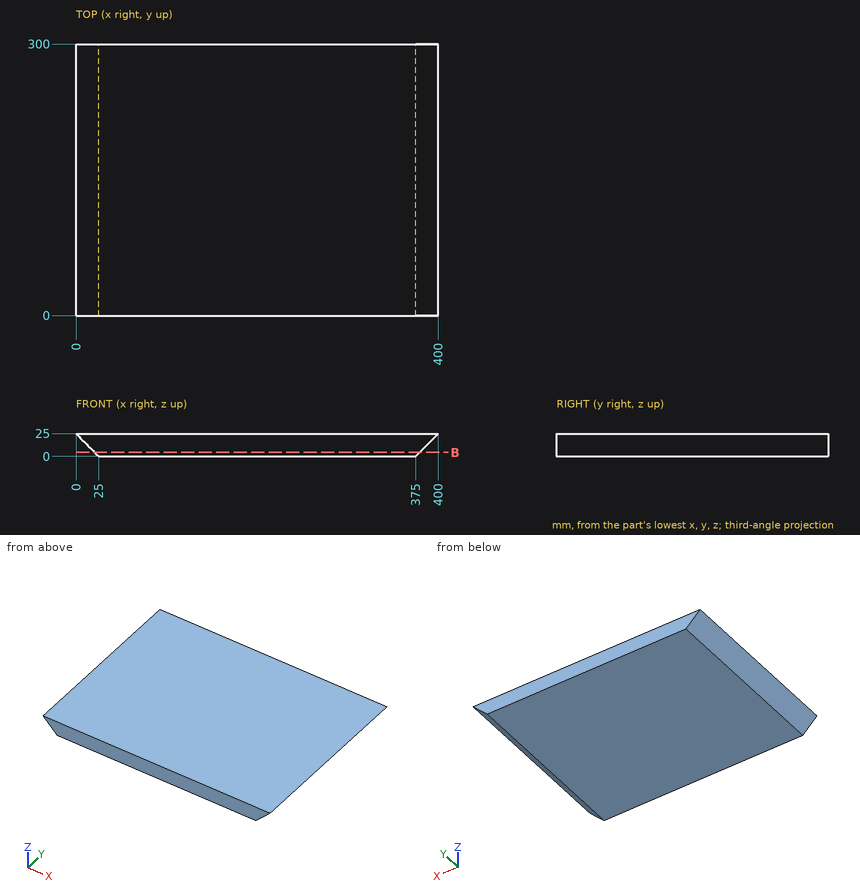
Could you check a few things on this drawing? It's one solid part, dimensions in mm from its lowest x, y, z. Give positions to 0.01 mm unless a question says otherwise; leave off trailing zeros. Order: outer loops, then holes, each group sorted by start corner. A loop starts at its lowest first (then second) coordinate and runs counter-clockwise, first axis right, second up. Notation, with made-up numbers: (5.5, 64) -> (34.5, 64) arc R19 cw to (34.5, 95) -> close; hole circle Ø7 at (79.5, 69). An arc over 180 degrees is marked (long way). Answer in a Markdown table with one row per item. Add a question column.
Item 1: I'm going to push flat-ended pins straight in: P1, Ø12, axis at x = 295, z = 7.5, coming from the -Y side; P2, Ø2, axis at y = 256, z = 22, coming from the -X side; P3, Ø4, axis at y = 242.5, z = 12, coming from the -X side. Where does each tip first touch, or does it pass through?
Item 2: Imagine slicing it at B-B (z = 4.5). List the corners of the cut face in (x, y) for me, and give its area (3 significant figures).
Item 3: Please list where these lines run through material, in increasing order: probe 1 along X at (y, z) = (228, 8.5); probe 2 along X at (y, z) = (145.5, 8.25).
Result:
| question | item | result |
|---|---|---|
| 1 | P1 | y = 0 |
| 1 | P2 | x = 2 |
| 1 | P3 | x = 11 |
| 2 | outline | (20.5, 0) -> (379.5, 0) -> (379.5, 300) -> (20.5, 300) -> close |
| 2 | area | 108,000 mm2 |
| 3 | probe 1 | 16.5 to 383.5 |
| 3 | probe 2 | 16.75 to 383.25 |
